```python
from build123d import *

# Parameters (mm, degrees)
F1_DEPTH = 25.4
F2_SCALE = 0.25


with BuildPart() as f1:
    # F0 (on Right) → F1 (new body)
    with BuildSketch(Plane.YZ):
        with BuildLine():
            ThreePointArc((-110.3992487095, 15.9628562986), (-108.4846328784, 12.1435644545), (-106.2483957789, 8.5032365015))
            Line((-106.2483957789, 8.5032365015), (-110.3992487095, 15.9628562986))
        make_face()
        with BuildLine():
            ThreePointArc((-24.1195932903, 64.1108403944), (-46.0880198127, 31.8647754474), (-40.4449835973, -6.7432109118))
            ThreePointArc((-40.4449835973, -6.7432109118), (-22.2285273136, 11.4155651853), (-15.5582582091, 36.2568199635))
            ThreePointArc((-15.5582582091, 36.2568199635), (-17.7468872986, 50.8268483826), (-24.1195932903, 64.1108403944))
        make_face()
        with BuildLine():
            Line((-52.4756349623, -88.1333723664), (37.4816562158, -23.9329912189))
            ThreePointArc((37.4816562158, -23.9329912189), (-5.3042368908, -32.6670185732), (-40.4449835973, -6.7432109118))
            ThreePointArc((-40.4449835973, -6.7432109118), (-76.3437133157, -12.0550910847), (-106.2483957789, 8.5032365015))
            Line((-106.2483957789, 8.5032365015), (-52.4756349623, -88.1333723664))
        make_face()
        with BuildLine():
            ThreePointArc((-106.2483957789, 8.5032365015), (-76.3437133157, -12.0550910847), (-40.4449835973, -6.7432109118))
            ThreePointArc((-40.4449835973, -6.7432109118), (-46.0880198127, 31.8647754474), (-24.1195932903, 64.1108403944))
            ThreePointArc((-24.1195932903, 64.1108403944), (-89.3162249481, 79.5619391689), (-110.3992487095, 15.9628562986))
            Line((-110.3992487095, 15.9628562986), (-106.2483957789, 8.5032365015))
        make_face()
        with BuildLine():
            ThreePointArc((-40.4449835973, -6.7432109118), (-5.3042368908, -32.6670185732), (37.4816562158, -23.9329912189))
            ThreePointArc((37.4816562158, -23.9329912189), (54.0392417852, -4.7941657865), (59.9991728249, 19.8011081666))
            ThreePointArc((59.9991728249, 19.8011081666), (31.3102321542, 67.3387752918), (-24.1195932903, 64.1108403944))
            ThreePointArc((-24.1195932903, 64.1108403944), (-17.7468872986, 50.8268483826), (-15.5582582091, 36.2568199635))
            ThreePointArc((-15.5582582091, 36.2568199635), (-22.2285273136, 11.4155651853), (-40.4449835973, -6.7432109118))
        make_face()
    extrude(amount=F1_DEPTH)


with BuildPart() as f1_1:
    # F2: moved
    add(f1.part.scale(F2_SCALE))


solid = f1_1.part
```
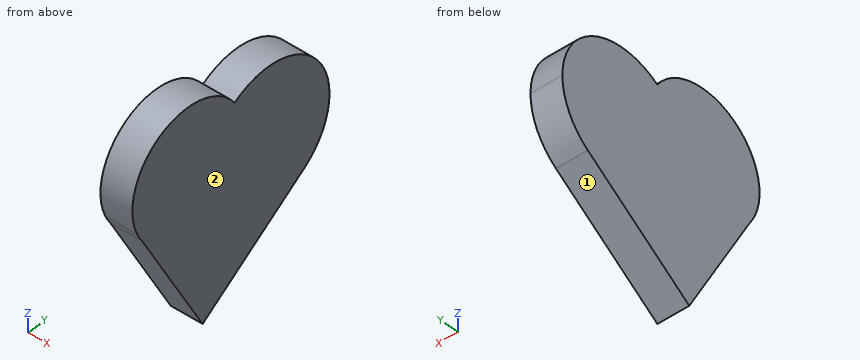
Work out the finished part from the listing and answer in its coordinate system (mm). Face numbers are marked on the shaded views. Coordinates: 2 decimals unless noted, no trailing zeros. Loops run counter-clockwise (first coordinate to the right, second up) from the corner with the lowest first, then second, coordinate; pieces in that order, holes last. Notation, with made-up numbers: (68, -7.75) - (95, -7.75) arc R18 cw to (95, 4.25) - close; hole circle Ø7 at (17, -4.5). An arc over 180 degrees is marked (long way). Use a Markdown table: item, result.
Item 1: Consider probe 1 along Y at (x, z) = (4.75, -19); probe 2 along Z at (x, y) = (2.75, -23.5); probe 3 along Y at (x, z) = (4.5, 15). Determine where each line is inside the solid, lowest interval first. Write a range as from..to.
Evaluation:
| item | result |
|---|---|
| probe 1 | y = -14.81..-8.87 |
| probe 2 | z = -3.38..19.15 |
| probe 3 | y = -27.17..10.48 |
Item 2: The mould has two halves that part along Z. Classify the marked faces 1 and 2: +Z half, -Z half, draft (parallel to the pull), parting line (faces both ways), or undercut.
Evaluation:
| item | result |
|---|---|
| face 1 | -Z half |
| face 2 | draft |
Item 3: Find section C-C, the plane x = 1.5. Determine the outline of the cut face in (y, z).
Evaluation:
| item | result |
|---|---|
| outline | (-26.56, 2.13) - (-13.12, -22.03) - (9.37, -5.98) arc R13.43 ccw to (-6.03, 16.03) arc R12.4 ccw to start |
Item 4: Given pin 1 Ø1 at (x, y) = (5.5, 0) entering from +Z; pin 2 Ø3 at (x, y) = (2.5, -23) entering from +Z, each flat-ended and moving along its own axis, determine where each tip first touches the part or whether it passes through.
Evaluation:
| item | result |
|---|---|
| pin 1 | stops at z = 18.34 |
| pin 2 | stops at z = 20.31 |
Item 5: Find section B-B, the plane y = -4. Determine the outline of the cut face in (x, z), and give its area (3 significant figures).
Evaluation:
| item | result |
|---|---|
| outline | (0, -15.53) - (6.35, -15.53) - (6.35, 17.17) - (0, 17.17) - close |
| area | 208 mm2 |
Item 6: Find section A-A, the plane z = 17. Determine the outline of the cut face in (x, y), and give its area (3 significant figures).
Evaluation:
| item | result |
|---|---|
| outline | (0, -25.81) - (6.35, -25.81) - (6.35, -6.76) - (0, -6.76) - close; (0, -4.37) - (6.35, -4.37) - (6.35, 7.5) - (0, 7.5) - close |
| area | 196 mm2 |
Item 7: Find section D-D, the plane z = -14.5. Determine the outline of the cut face in (x, y), and give its area (3 significant figures).
Evaluation:
| item | result |
|---|---|
| outline | (0, -17.31) - (6.35, -17.31) - (6.35, -2.56) - (0, -2.56) - close |
| area | 93.6 mm2 |
